Here's how the part is built. I have some questions about the finished solid (model axes, mm). Face numbers are marked on the shaded views. A direction names the side the tool comes from. Round coordinates to 2 decimals unless told otherwise and drop trailing zeros. Write each loop counter-clockwise with the first axis right and the second up, starting at its lowest first coordinate (ties: lowest second). Pieces come first, ordered by that corner, then holes. Notation, with made-up numbers: (40.25, -18) - (47.25, -18) arc R16 cw to (47.25, -10) - close; hole circle Ø4 at (-4.5, 7.5). An arc over 180 degrees is marked (long way). One line per item, written item: value. Start each with the question number.
Item 1: Imagine slicing it at B-B, the plane x = 13.5. Please give me the cut outline in (y, z) (1 decimal).
Item 2: If I drill on line 1 (Y direction, x = 21, z = 15); line 2 (Y direction, x = 13.5, z = 15); line 3 (Y direction, x = 18.5, z = 4.75), over which ranges is the centre line in solid material (lowest first)?
Item 3: Imagine slicing it at D-D, the plane x = 26. Please give me the cut outline in (y, z) (1 decimal), then the cut area to 3 significant figures.
Item 4: Thinking about a two-plate mould opening in Z: for the marked faces 3, 4 and 5, which applies, released by +Z, released by -Z, zero draft, split by the parting line, or undercut?
Item 5: Imagine slicing it at C-C, the plane z = 7.25. Please give me the cut outline in (x, y).
Item 6: For the marked faces 1 and 2, which set-ups out of +Z, -Z, +X, -X, +Y, -Y let a thin tool reach every point of the face, with its end or its side?
Item 7: Imagine slicing it at A-A, the plane y = 10. Please give me the cut outline in (x, z), then the cut area to 3 significant figures.
Autodesk Inventor part; units mm, degrees
ref_plane "YZ Plane" through (0, 0, 0) normal (1, 0, 0) x (0, 1, 0)
ref_plane "XZ Plane" through (0, 0, 0) normal (0, 1, 0) x (-1, 0, 0)
ref_plane "XY Plane" through (0, 0, 0) normal (0, 0, 1) x (1, 0, 0)
sketch "Sketch1" plane through (0, 0, 0) normal (0, 0, 1) x (1, 0, 0)
  line L0 (0, 0) -> (41, 0)
  line L1 (41, 0) -> (41, 61.3)
  line L2 (41, 61.3) -> (0, 61.3)
  line L3 (0, 61.3) -> (0, 0)
  dimension "d0" = 61.3
  dimension "d1" = 41
extrude "Extrusion1" add sketch "Sketch1" along normal blind 30
sketch "Sketch2" plane through (0, 0, 0) normal (-1, 0, 0) x (0, 0, 1)
  circle A0 centre (15, 10) radius 1.5875
  line L0 (0, 0) -> (30, 0)
  line L1 (0, 61.3) -> (0, 0)
  dimension "d4" = 3.175
  dimension "d5" = 10
  dimension "d6" = 15
extrude "Extrusion2" cut sketch "Sketch2" against normal through all
sketch "Sketch3" plane through (0, 61.3, 0) normal (0, 1, 0) x (1, 0, 0)
  line L0 (0, 0) -> (0, -30)
  line L1 (41, 0) -> (41, -30)
  line L2 (0, 0) -> (41, 0)
  line L3 (41, 0) -> (41, -30)
  line L4 (41, -30) -> (0, -30)
  line L5 (0, -30) -> (0, 0)
  circle A0 centre (26, -15) radius 10
  dimension "d9" = 15
  dimension "d10" = 15
  dimension "d11" = 20
extrude "Extrusion3" cut sketch "Sketch3" against normal blind 10
properties part number "SolidnoidV"
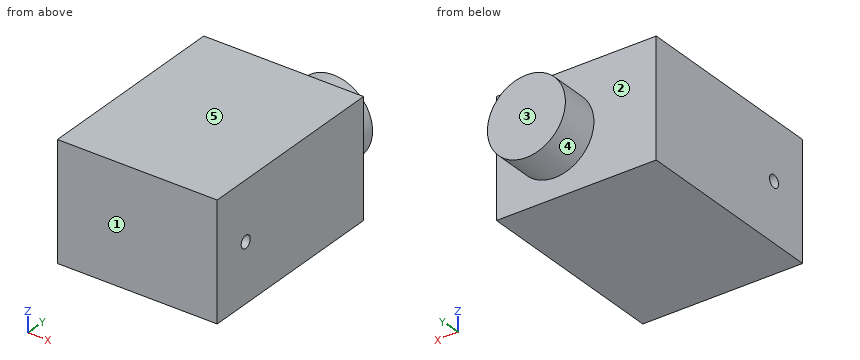
Values follow:
1. outline: (0, 0) - (51.3, 0) - (51.3, 30) - (0, 30) - close; hole circle Ø3.2 at (10, 15)
2. line 1: y = 0 to 8.41, 11.59 to 61.3
2. line 2: y = 0 to 8.41, 11.59 to 51.3
2. line 3: y = 0 to 51.3
3. outline: (0, 0) - (51.3, 0) - (51.3, 5) - (61.3, 5) - (61.3, 25) - (51.3, 25) - (51.3, 30) - (0, 30) - close; hole circle Ø3.2 at (10, 15)
3. area: 1,730 mm^2
4. face 3: zero draft
4. face 4: split by the parting line
4. face 5: released by +Z
5. outline: (0, 0) - (41, 0) - (41, 51.3) - (32.32, 51.3) - (32.32, 61.3) - (19.68, 61.3) - (19.68, 51.3) - (0, 51.3) - close
6. face 1: +Z, -Z, +X, -X, -Y
6. face 2: +Y
7. outline: (0, 0) - (41, 0) - (41, 13.41) - (0, 13.41) - close; (0, 16.59) - (41, 16.59) - (41, 30) - (0, 30) - close
7. area: 1,100 mm^2
